Check sheet for the modelled part. Datum: model origin and axes. Units: mm. Face numbers are marked on the shaded views. A direction names the side the tool comes from. Give positions to 0.01 mm unless a question says otherwise; leave off trailing zeros. Write each loop counter-clockwise with the first axis right and the second up, starting at its lowest first coordinate (ties: lowest second). Pieces come first, ordered by that corner, then holes.
from build123d import *

# Parameters (mm, degrees)
SKETCH1_R           = 6
BOSS_EXTRUDE1_DEPTH = 36
BOSS_EXTRUDE2_DEPTH = 8
SKETCH3_OUTSIDE_W   = 53.532
SKETCH3_OUTSIDE_H   = 51.488
SKETCH3_OUTSIDE_R   = 9.5
CUT_EXTRUDE1_DEPTH  = 8
CUT_EXTRUDE1_DRAFT  = -50
SKETCH4_OUTSIDE_W   = 53.532
SKETCH4_OUTSIDE_H   = 51.488
SKETCH4_OUTSIDE_R   = 9.5
CUT_EXTRUDE3_DEPTH  = 8
CUT_EXTRUDE3_DRAFT  = -50
BOSS_EXTRUDE3_DEPTH = 8
SKETCH6_OUTSIDE_W   = 54.894
SKETCH6_OUTSIDE_H   = 52.85
SKETCH6_OUTSIDE_R   = 9.5
CUT_EXTRUDE6_DEPTH  = 8
CUT_EXTRUDE6_DRAFT  = -50
SKETCH7_OUTSIDE_W   = 54.894
SKETCH7_OUTSIDE_H   = 52.85
SKETCH7_OUTSIDE_R   = 9.481063721
CUT_EXTRUDE7_DEPTH  = 8
CUT_EXTRUDE7_DRAFT  = -50
SKETCH8_R           = 6
SKETCH8_R_2         = 5
CUT_EXTRUDE8_DEPTH  = 36


with BuildPart() as part:
    # Sketch1 → Boss-Extrude1 (new body)
    with BuildSketch(Plane.XY):
        Circle(SKETCH1_R)
    extrude(amount=BOSS_EXTRUDE1_DEPTH)

    # Sketch2 → Boss-Extrude2 (add)
    with BuildSketch(Plane(origin=(0, 0, 0), x_dir=(-1, 0, 0), z_dir=(0, 0, -1))):
        Polygon((-10.93381737, 0.885985919), (-6.234194998, -9.025970644), (4.699622372, -9.911956562), (10.93381737, -0.885985919), (6.234194998, 9.025970644), (-4.699622372, 9.911956562), align=None)
    extrude(amount=BOSS_EXTRUDE2_DEPTH)


with BuildPart() as cut_extrude1_tool:
    # Sketch3 outside → Cut-Extrude1 (with draft: the straight prism first)
    with BuildSketch(Plane.XY):
        Rectangle(SKETCH3_OUTSIDE_W, SKETCH3_OUTSIDE_H)
        Circle(SKETCH3_OUTSIDE_R, mode=Mode.SUBTRACT)
    extrude(amount=-CUT_EXTRUDE1_DEPTH)
    # Cut-Extrude1: the draft: its side faces are tilted about the plane it starts from
    cut_extrude1_sides = [cut_extrude1_tool.faces().sort_by_distance(p)[0] for p in [
        (0, -25.744, -4),
        (26.766, 0, -4),
        (0, 25.744, -4),
        (-26.766, 0, -4),
        (-9.5, 0, -4),
    ]]
    draft(cut_extrude1_sides, Plane.XY, CUT_EXTRUDE1_DRAFT)


with BuildPart() as part_1:
    add(part.part)

    # Cut-Extrude1: cut by cut_extrude1_tool
    add(cut_extrude1_tool.part, mode=Mode.SUBTRACT)


with BuildPart() as cut_extrude3_tool:
    # Sketch4 outside → Cut-Extrude3 (with draft: the straight prism first)
    with BuildSketch(Plane(origin=(0, 0, -8), x_dir=(-1, 0, 0), z_dir=(0, 0, -1))):
        Rectangle(SKETCH4_OUTSIDE_W, SKETCH4_OUTSIDE_H)
        Circle(SKETCH4_OUTSIDE_R, mode=Mode.SUBTRACT)
    extrude(amount=-CUT_EXTRUDE3_DEPTH)
    # Cut-Extrude3: the draft: its side faces are tilted about the plane it starts from
    cut_extrude3_sides = [cut_extrude3_tool.faces().sort_by_distance(p)[0] for p in [
        (0, -25.744, -4),
        (-26.766, 0, -4),
        (0, 25.744, -4),
        (26.766, 0, -4),
        (9.5, 0, -4),
    ]]
    draft(cut_extrude3_sides, Plane(origin=(0, 0, -8), x_dir=(-1, 0, 0), z_dir=(0, 0, -1)), CUT_EXTRUDE3_DRAFT)


with BuildPart() as part_2:
    add(part_1.part)

    # Cut-Extrude3: cut by cut_extrude3_tool
    add(cut_extrude3_tool.part, mode=Mode.SUBTRACT)

    # Sketch5 → Boss-Extrude3 (add)
    with BuildSketch(Plane.XY.offset(36)):
        Polygon((-6.252986911, 8.986336688), (-10.908889314, -0.92207717), (-4.655902404, -9.908413858), (6.252986911, -8.986336688), (10.908889314, 0.92207717), (4.655902404, 9.908413858), align=None)
    extrude(amount=BOSS_EXTRUDE3_DEPTH)


with BuildPart() as cut_extrude6_tool:
    # Sketch6 outside → Cut-Extrude6 (with draft: the straight prism first)
    with BuildSketch(Plane(origin=(0, 0, 36), x_dir=(-1, 0, 0), z_dir=(0, 0, -1))):
        Rectangle(SKETCH6_OUTSIDE_W, SKETCH6_OUTSIDE_H)
        Circle(SKETCH6_OUTSIDE_R, mode=Mode.SUBTRACT)
    extrude(amount=-CUT_EXTRUDE6_DEPTH)
    # Cut-Extrude6: the draft: its side faces are tilted about the plane it starts from
    cut_extrude6_sides = [cut_extrude6_tool.faces().sort_by_distance(p)[0] for p in [
        (0, -26.425, 40),
        (-27.447, 0, 40),
        (0, 26.425, 40),
        (27.447, 0, 40),
        (9.5, 0, 40),
    ]]
    draft(cut_extrude6_sides, Plane(origin=(0, 0, 36), x_dir=(-1, 0, 0), z_dir=(0, 0, -1)), CUT_EXTRUDE6_DRAFT)


with BuildPart() as part_3:
    add(part_2.part)

    # Cut-Extrude6: cut by cut_extrude6_tool
    add(cut_extrude6_tool.part, mode=Mode.SUBTRACT)


with BuildPart() as cut_extrude7_tool:
    # Sketch7 outside → Cut-Extrude7 (with draft: the straight prism first)
    with BuildSketch(Plane.XY.offset(44)):
        Rectangle(SKETCH7_OUTSIDE_W, SKETCH7_OUTSIDE_H)
        Circle(SKETCH7_OUTSIDE_R, mode=Mode.SUBTRACT)
    extrude(amount=-CUT_EXTRUDE7_DEPTH)
    # Cut-Extrude7: the draft: its side faces are tilted about the plane it starts from
    cut_extrude7_sides = [cut_extrude7_tool.faces().sort_by_distance(p)[0] for p in [
        (0, -26.425, 40),
        (27.447, 0, 40),
        (0, 26.425, 40),
        (-27.447, 0, 40),
        (-9.481063721, 0, 40),
    ]]
    draft(cut_extrude7_sides, Plane.XY.offset(44), CUT_EXTRUDE7_DRAFT)


with BuildPart() as part_4:
    add(part_3.part)

    # Cut-Extrude7: cut by cut_extrude7_tool
    add(cut_extrude7_tool.part, mode=Mode.SUBTRACT)

    # Sketch8 → Cut-Extrude8 (cut)
    with BuildSketch(Plane.XY):
        Circle(SKETCH8_R)
        Circle(SKETCH8_R_2, mode=Mode.SUBTRACT)
    extrude(amount=CUT_EXTRUDE8_DEPTH, mode=Mode.SUBTRACT)


solid = part_4.part
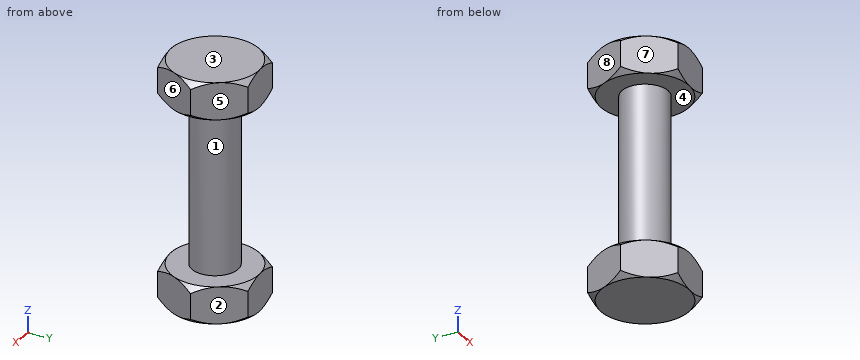
1) Sectioned sample at B-B on y = 0. Record the boundary of the cut face in (x, z), then the cut area to 3 significant figures.
2) Scan lines: L1, parallel to Z at x = -5.75, y = 4; L2, parallel to X at y = 1, z = -1; L3, parallel to X at y = -1, z = 9.5. Record each from-to range of solid material in increasing order.
3) Sectioned sample at A-A on z = 41.5. Record the boundary of the cut face in (x, y).
4) Sectioned sample at C-C on z = 33. Record the boundary of the cut face in (x, y), then the cut area to 3 significant figures.
5) Draft check along Z on the marked faces 1, 2 and 3. Enter one of: +Z half, -Z half, draft (parallel to the pull), parting line (faces both ways), or undercut.
6) Access from +Z, -Z, +X, -X, +Y, -Y to the whole of each face (thin tool, end or side, straight path). Record for the marked faces 4, 5, 6, 7 and 8.
7) Gauge pin test, flat ends, axial feed: pin 1 (5 mm diameter, centred on x = 6, z = 16, fed in from -Y); pin 2 (1.5 mm diameter, centred on y = -3.5, z = 11.5, fed in from -X); pin 3 (6 mm diameter, centred on x = -1, z = 19, fed in from -Y). Record the tip position at first contact, or that the pin passes through.
Answers below:
1. outline: (-10.51, -7.15) - (-9.5, -8) - (9.5, -8) - (10.51, -7.15) - (10.51, -0.85) - (9.5, 0) - (5, 0) - (5, 36) - (9.5, 36) - (10.48, 36.82) - (10.48, 43.17) - (9.48, 44) - (-9.48, 44) - (-10.48, 43.17) - (-10.48, 36.82) - (-9.5, 36) - (-5, 36) - (-5, 0) - (-9.5, 0) - (-10.51, -0.85) - close
1. area: 692 mm2
2. L1: z = -8 to 0, 36 to 44
2. L2: x = -10.04 to 10.64
2. L3: x = -4.9 to 4.9
3. outline: (-10.91, -0.92) - (-4.66, -9.91) - (6.25, -8.99) - (10.91, 0.92) - (4.66, 9.91) - (-6.25, 8.99) - close
4. outline: circle Ø10 at (0, 0)
4. area: 78.5 mm2
5. face 1: undercut
5. face 2: draft
5. face 3: +Z half
6. face 4: none
6. face 5: +Z, +X, +Y
6. face 6: +Z, +X, -Y
6. face 7: +Z, -X, -Y
6. face 8: +Z, -X, +Y
7. pin 1: stops at y = -3.57
7. pin 2: stops at x = -4.18
7. pin 3: stops at y = -5
